Part model, mm, in its own coordinate system. A direction names the side the tool comes from. Round coordinates to 2 decimals unless told otherwise and drop trailing zeros. Loops run counter-clockwise (first coordinate to the right, second up) from the corner with the lowest first, then second, coordinate; pieces in that order, holes last.
(1) Cut at B-B on y = -6.5. List the corners of the cut face in (x, z), then the cut area to 3 significant figures.
(2) Mould opens along Y. For faces 1 (the face through (0, 70, 4)), 2 (the face through (-2, 1, 8)), 3 (the face through (-50, -58, 4)) say: +Y half, -Y half, draft (parallel to the pull), parting line (faces both ways), or undercut.
(3) Cut at C-C on z = 4.25. Count the separate pieces of the cut face and the enclosed holes in it, then the cut area to 3 significant figures.
(4) Cut at A-A on y = 90. List the corners of the cut face in (x, z).
(5) Cut at D-D on y = 64. List the corners of the cut face in (x, z), then the cut area to 3 significant figures.
(6) Flat gauge pin, fed straight in: pin 1 (2.5 mm diameter, centred on y = -75, z = 4.5, fed in from -X) (3 decimals). Where does the tip first touch, or does it go through?
(7) Tool access for faces 4 (the face through (47, -45, 4)), 5 (the face through (69, 100, 4)), 6 (the face through (-160, 0, 4)), 7 (the face through (28, -75, 4)): list every direction of +Z, -Z, +X, -X, +Y, -Y with a clear straight run to the whole face (end or side of a thin tool).
(8) Probe probe 1 along X at (y, z) = (-3, 5.75); probe 2 along X at (y, z) = (-38.5, 5.5); probe 3 along Y at (x, z) = (92.8, 4). List the from-to ranges inside material, lowest first.
Autodesk Inventor part; units mm, degrees
ref_plane "YZ Plane" through (0, 0, 0) normal (1, 0, 0) x (0, 1, 0)
ref_plane "XZ Plane" through (0, 0, 0) normal (0, 1, 0) x (-1, 0, 0)
ref_plane "XY Plane" through (0, 0, 0) normal (0, 0, 1) x (1, 0, 0)
sketch "Esquisse1" plane through (0, 0, 0) normal (0, 0, 1) x (1, 0, 0)
  line L0 (-170, -60) -> (-170, 60)
  line L1 (170, 60) -> (170, -60)
  line L2 (170, -100) -> (-170, 100) construction
  line L3 (-170, -100) -> (170, 100) construction
  line L4 (-90, 100) -> (-170, 60)
  line L5 (90, 100) -> (170, 60)
  line L6 (-170, -60) -> (-110, -100)
  line L7 (110, -100) -> (170, -60)
  line L8 (48, 100) -> (90, 100)
  line L9 (52, 0) -> (-69, 0)
  line L10 (28, -80) -> (28, -70)
  line L11 (28, -70) -> (-28, -70)
  line L12 (-28, -70) -> (-28, -80)
  line L13 (-28, -80) -> (-48, -100)
  line L14 (28, -80) -> (48, -100)
  line L15 (110, -100) -> (48, -100)
  line L16 (-48, -100) -> (-110, -100)
  line L17 (-28, 70) -> (-28, 80)
  line L18 (-28, 80) -> (-48, 100)
  line L19 (28, 70) -> (-28, 70)
  line L20 (28, 80) -> (28, 70)
  line L21 (28, 80) -> (48, 100)
  line L22 (-90, 100) -> (-48, 100)
  line L23 (48, 100) -> (90, 100)
  point P0 (0, 0)
  dimension "d2" = 80
  dimension "d3" = 40
  dimension "d4" = 80
  dimension "d5" = 40
  dimension "d6" = 40
  dimension "d7" = 60
  dimension "d8" = 60
  dimension "d9" = 40
extrude "Plaque" add sketch "Esquisse1" along normal blind 8
sketch "Esquisse2" plane through (0, 0, 8) normal (0, 0, 1) x (1, 0, 0)
  circle A0 centre (-146, 35) radius 2
  circle A1 centre (-132, 35) radius 2
  circle A2 centre (-146, -35) radius 2
  circle A3 centre (-132, -35) radius 2
  line L0 (-170, 60) -> (-170, -60)
  line L1 (0, 25.5561) -> (0, -26.1527)
  circle A4 centre (146, 35) radius 2
  circle A5 centre (132, 35) radius 2
  circle A6 centre (146, -35) radius 2
  circle A7 centre (132, -35) radius 2
  point P0 (0, 0)
  dimension "d12" = 4
  dimension "d13" = 4
  dimension "d14" = 4
  dimension "d15" = 4
  dimension "d16" = 14
  dimension "d17" = 14
  dimension "d18" = 24
  dimension "d19" = 24
  dimension "d20" = 35
  dimension "d21" = 35
  dimension "d22" = 35
  dimension "d23" = 35
hole "Fixation_Encodeur" at (-132, 35, 8) at (-146, 35, 8) at (-146, -35, 8) at (-132, -35, 8) at (132, 35, 8) at (146, 35, 8) at (146, -35, 8) at (132, -35, 8) direction (0, 0, -1) diameter 4 end through all
sketch "Esquisse3" plane through (0, 0, 8) normal (0, 0, 1) x (1, 0, 0)
  line L0 (-140.5, -19) -> (-100.5, -19)
  line L1 (-100.5, -19) -> (-100.5, 19)
  line L2 (-100.5, 19) -> (-140.5, 19)
  line L3 (-140.5, 19) -> (-140.5, -19)
  line L4 (-140.5, -19) -> (-100.5, 19) construction
  line L5 (-100.5, -19) -> (-140.5, 19) construction
  line L6 (-90, 100) -> (-170, 60)
  line L7 (-170, 60) -> (-170, -60)
  line L8 (-170, -60) -> (-110, -100)
  line L9 (48, -100) -> (110, -100)
  line L10 (110, -100) -> (170, -60)
  line L11 (170, -60) -> (170, 60)
  line L12 (170, 60) -> (90, 100)
  line L13 (-48, 100) -> (-90, 100)
  line L14 (0, 102.1518) -> (0, -90)
  line L15 (140.5, -19) -> (100.5, -19)
  line L16 (100.5, -19) -> (100.5, 19)
  line L17 (100.5, 19) -> (140.5, 19)
  line L18 (140.5, 19) -> (140.5, -19)
  line L19 (140.5, -19) -> (100.5, 19) construction
  line L20 (100.5, -19) -> (140.5, 19) construction
  line L21 (-110, -100) -> (-48, -100)
  line L22 (-48, -100) -> (-28, -80)
  line L23 (-28, -80) -> (-28, -70)
  line L24 (-28, -70) -> (28, -70)
  line L25 (28, -70) -> (28, -80)
  line L26 (28, -80) -> (48, -100)
  line L27 (90, 100) -> (48, 100)
  line L28 (48, 100) -> (28, 80)
  line L29 (28, 80) -> (28, 70)
  line L30 (28, 70) -> (-28, 70)
  line L31 (-28, 70) -> (-28, 80)
  line L32 (-28, 80) -> (-48, 100)
  point P0 (0, 0)
  point P1 (-120.5, 0)
  point P2 (120.5, 0)
  dimension "d31" = 29.5
  dimension "d32" = 40
  dimension "d33" = 38
  dimension "d53" = 19
hole "Fixation_Moteur" at (-140.5, 19, 8) at (-100.5, 19, 8) at (-100.5, -19, 8) at (-140.5, -19, 8) at (140.5, 19, 8) at (140.5, -19, 8) at (100.5, 19, 8) at (100.5, -19, 8) direction (0, 0, -1) diameter 4 end through all
sketch "Esquisse4" plane through (0, 0, 8) normal (0, 0, 1) x (1, 0, 0)
  line L0 (-60, -25) -> (-40, -25)
  line L1 (-60, 25) -> (-60, -25)
  line L2 (-60, -25) -> (-39.915, 7.067) construction
  circle A0 centre (100.5, 19) radius 2
  circle A1 centre (140.5, 19) radius 2
  circle A2 centre (-100.5, -19) radius 2
  circle A3 centre (-140.5, 19) radius 2
  circle A4 centre (-100.5, 19) radius 2
  circle A5 centre (-140.5, -19) radius 2
  circle A6 centre (140.5, -19) radius 2
  circle A7 centre (100.5, -19) radius 2
  line L3 (-90, 100) -> (-170, 60)
  line L4 (-170, 60) -> (-170, -60)
  line L5 (-170, -60) -> (-110, -100)
  line L6 (48, -100) -> (110, -100)
  line L7 (110, -100) -> (170, -60)
  line L8 (170, -60) -> (170, 60)
  line L9 (170, 60) -> (90, 100)
  line L10 (-48, 100) -> (-90, 100)
  line L11 (40, 25) -> (60, 25)
  line L12 (60, 25) -> (60, -25)
  line L13 (60, -25) -> (40, -10.6364) construction
  line L14 (40, 25) -> (40, -25)
  line L15 (-40, -25) -> (-40, 25)
  line L16 (-40, 25) -> (-60, 25)
  line L17 (-39.915, 7.067) -> (-60, 25) construction
  line L18 (40, 10.0232) -> (60, 25) construction
  line L19 (60, -25) -> (40, -25)
  line L20 (-110, -100) -> (-48, -100)
  line L21 (-48, -100) -> (-28, -80)
  line L22 (-28, -80) -> (-28, -70)
  line L23 (-28, -70) -> (28, -70)
  line L24 (28, -70) -> (28, -80)
  line L25 (28, -80) -> (48, -100)
  line L26 (90, 100) -> (48, 100)
  line L27 (48, 100) -> (28, 80)
  line L28 (28, 80) -> (28, 70)
  line L29 (28, 70) -> (-28, 70)
  line L30 (-28, 70) -> (-28, 80)
  line L31 (-28, 80) -> (-48, 100)
  point P0 (-39.915, 7.067)
  dimension "d50" = 110
  dimension "d157" = 110
  dimension "d158" = 20
  dimension "d159" = 20
extrude "Passage_Courroie" cut sketch "Esquisse4" against normal up to surface (8 mm away) contours L1 L16 L15 L0 | L11 L12 L19 L14
sketch "Esquisse5" plane through (0, 0, 8) normal (0, 0, 1) x (1, 0, 0)
  line L0 (0, 30.4597) -> (0, -30.4597)
  line L1 (-17.5456, 0) -> (17.5456, 0)
  line L2 (-80, 40) -> (-80, -40)
  line L3 (-80, -40) -> (-110, -40)
  line L4 (-110, 30) -> (-110, 40)
  line L5 (-110, 40) -> (-80, 40)
  line L6 (-88, 90) -> (-142, 63)
  line L7 (-142, 63) -> (-142, 30)
  line L8 (-142, 30) -> (-110, 30)
  line L9 (-110, -30) -> (-142, -30)
  line L10 (-142, -30) -> (-142, -63)
  line L11 (-142, -63) -> (-102, -90)
  line L12 (-102, -90) -> (-44, -90)
  line L13 (-44, -90) -> (-34, -80)
  line L14 (-34, -80) -> (-34, 80)
  line L15 (-34, 80) -> (-44, 90)
  line L16 (-44, 90) -> (-88, 90)
  line L17 (-110, -40) -> (-110, -30)
  circle A0 centre (-134, -35) radius 2
  circle A1 centre (-134, 35) radius 2
  circle A2 centre (-120, 35) radius 2
  circle A3 centre (-120, -35) radius 2
  line L18 (-88, 90) -> (-142, 63)
  line L19 (-142, 63) -> (-142, 30)
  line L20 (-142, 30) -> (-110, 30)
  line L21 (-110, 30) -> (-110, 40)
  line L22 (-110, 40) -> (-80, 40)
  line L23 (-80, 40) -> (-80, -40)
  line L24 (-80, -40) -> (-110, -40)
  line L25 (-110, -40) -> (-110, -30)
  line L26 (-110, -30) -> (-142, -30)
  line L27 (-142, -30) -> (-142, -63)
  line L28 (-142, -63) -> (-102, -90)
  line L29 (-102, -90) -> (-44, -90)
  line L30 (-44, -90) -> (-34, -80)
  line L31 (-34, -80) -> (-34, 80)
  line L32 (-34, 80) -> (-44, 90)
  line L33 (-44, 90) -> (-88, 90)
  line L34 (-138, 53.1115) -> (-96.2229, 74)
  line L35 (-96.2229, 74) -> (-62, 74)
  line L36 (-62, 74) -> (-62, -74)
  line L37 (-62, -74) -> (-109.1054, -74)
  line L38 (-109.1054, -74) -> (-138, -54.4961)
  line L39 (96.2229, 74) -> (62, 74)
  line L40 (138, 53.1115) -> (96.2229, 74)
  line L41 (62, -74) -> (109.1054, -74)
  line L42 (109.1054, -74) -> (138, -54.4961)
  line L43 (-170, 60) -> (-170, -60)
  point P0 (0, 0)
  point P1 (72.8, -55)
  point P2 (92.8, -55)
  point P3 (112.8, -55)
  point P4 (-72.8, -55)
  point P5 (-92.8, -55)
  point P6 (-112.8, -55)
  point P7 (72.8, 55)
  point P8 (92.8, 55)
  point P9 (112.8, 55)
  point P10 (-72.8, 55)
  point P11 (-92.8, 55)
  point P12 (-112.8, 55)
  point P13 (0, 0)
  dimension "d174" = 10.6334
  dimension "d175" = 47.1054
  dimension "d176" = 34.2229
  dimension "d177" = 41.7771
  dimension "d178" = 28.8946
  dimension "d179" = 32
  dimension "d180" = 32
  dimension "d198" = 55
  dimension "d199" = 55
  dimension "d200" = 55
hole "Fixation_Base" at (72.8, -55, 8) at (92.8, -55, 8) at (112.8, -55, 8) at (-112.8, 55, 8) at (-72.8, 55, 8) at (-92.8, 55, 8) at (-112.8, -55, 8) at (-92.8, -55, 8) at (-72.8, -55, 8) at (72.8, 55, 8) at (92.8, 55, 8) at (112.8, 55, 8) at (138, 53.1115, 8) at (62, 74, 8) at (138, -54.4961, 8) at (62, -74, 8) at (-62, -74, 8) at (-138, -54.4961, 8) at (-138, 53.1115, 8) at (-62, 74, 8) direction (0, 0, -1) diameter 6 end through all
sketch "Esquisse7" plane through (0, 0, 8) normal (0, 0, 1) x (1, 0, 0)
  line L0 (-54, 90) -> (54, 90)
  line L1 (-156, 0) -> (156, 0)
  line L2 (-170, 60) -> (-170, -60)
  line L3 (170, -60) -> (170, 60)
  line L4 (-110, -100) -> (110, -100)
  line L5 (-48, 100) -> (-90, 100)
  line L6 (-156, 0) -> (-156, 51.3475)
  line L7 (-156, 0) -> (-156, -52.5074)
  line L8 (156, 0) -> (156, 51.3475)
  line L9 (156, 0) -> (156, -52.5074)
  line L10 (-90, 100) -> (-170, 60)
  line L11 (170, 60) -> (90, 100)
  line L12 (110, -100) -> (170, -60)
  line L13 (-170, -60) -> (-110, -100)
  point P0 (0, 0)
  point P1 (-54, -90)
  point P2 (54, -90)
  dimension "d88" = 14
  dimension "d89" = 14
  dimension "d93" = 10
  dimension "d94" = 108
  dimension "d95" = 54
  dimension "d123" = 108
  dimension "d124" = 10
  dimension "d125" = 10
  dimension "d126" = 56
  dimension "d160" = 56
  dimension "d181" = 14
  dimension "d182" = 14
  dimension "d186" = 14
  dimension "d187" = 14
hole "Fixation_Etage3" at (-54, 90, 8) at (-54, -90, 8) at (54, -90, 8) at (54, 90, 8) at (-156, 51.3475, 8) at (-156, -52.5074, 8) at (156, 51.3475, 8) at (156, -52.5074, 8) direction (0, 0, -1) diameter 8 end through all
sketch "Esquisse8" plane through (0, 0, 8) normal (0, 0, 1) x (1, 0, 0)
  line L0 (-160, -25) -> (-170, -25)
  line L1 (-170, -25) -> (-170, 25)
  line L2 (-170, 25) -> (-160, 25)
  line L3 (-160, 25) -> (-160, -25)
  line L4 (-160, -25) -> (-170, 25) construction
  line L5 (-170, -25) -> (-160, 25) construction
  line L6 (0, 43.7993) -> (0, -83.0015)
  line L7 (160, -25) -> (170, -25)
  line L8 (170, -25) -> (170, 25)
  line L9 (170, 25) -> (160, 25)
  line L10 (160, 25) -> (160, -25)
  line L11 (160, -25) -> (170, 25) construction
  line L12 (170, -25) -> (160, 25) construction
  point P0 (0, 0)
  point P1 (-165, 0)
  point P2 (165, 0)
  dimension "d106" = 50
  dimension "d107" = 10
  dimension "d108" = 160
  dimension "d191" = 25
extrude "Passage_Encodeur" cut sketch "Esquisse8" against normal up to surface (8 mm away)
chamfer "Chanfrein1" distance 10 angle 45 4 edges at (-160, 25, 4) (-160, -25, 4) (160, 25, 4) (160, -25, 4)
sketch "Esquisse10" plane through (0, 0, 8) normal (0, 0, 1) x (1, 0, 0)
  line L0 (-50, -35) -> (-50, -55) construction
  line L1 (-53, -35) -> (-53, -55)
  line L2 (-47, -55) -> (-47, -35)
  arc A0 (-47, -35) -> (-53, -35) centre (-50, -35) ccw
  arc A1 (-53, -55) -> (-47, -55) centre (-50, -55) ccw
  line L3 (-40, -25) -> (-60, -25)
  point P0 (0, 0)
  point P1 (-50, -45)
  dimension "d192" = 10
  dimension "d193" = 20
  dimension "d194" = 3
  dimension "d195" = 10
extrude "Extrusion4" cut sketch "Esquisse10" against normal blind 10
mirror "Symétrie1" about plane through (0, 0, 0) normal (1, 0, 0) of "Extrusion4"
properties part number "Support_Moteur"
Final values:
1. outline: (-160, 0) - (-60, 0) - (-60, 8) - (-160, 8) - close; (-40, 0) - (40, 0) - (40, 8) - (-40, 8) - close; (60, 0) - (160, 0) - (160, 8) - (60, 8) - close
1. area: 2,240 mm2
2. face 1: +Y half
2. face 2: draft
2. face 3: undercut
3. separate pieces: 1
3. enclosed holes: 48
3. area: 54,000 mm2
4. outline: (-110, 0) - (-58, 0) - (-58, 8) - (-110, 8) - close; (-50, 0) - (-38, 0) - (-38, 8) - (-50, 8) - close; (38, 0) - (50, 0) - (50, 8) - (38, 8) - close; (58, 0) - (110, 0) - (110, 8) - (58, 8) - close
5. outline: (-162, 0) - (162, 0) - (162, 8) - (-162, 8) - close
5. area: 2,590 mm2
6. pin 1: stops at x = -149.375
7. face 4: +Z, -Z
7. face 5: +Z, -Z, +X, -X, +Y
7. face 6: +Z, -Z, -X
7. face 7: +Z, -Z, -Y
8. probe 1: x = -160 to -60, -40 to 40, 60 to 160
8. probe 2: x = -170 to -53, -47 to 47, 53 to 170
8. probe 3: y = -100 to -58, -52 to 52, 58 to 98.6
